Autodesk Inventor part; units mm, degrees
ref_plane "YZ Plane" through (0, 0, 0) normal (1, 0, 0) x (0, 1, 0)
ref_plane "XZ Plane" through (0, 0, 0) normal (0, 1, 0) x (-1, 0, 0)
ref_plane "XY Plane" through (0, 0, 0) normal (0, 0, 1) x (1, 0, 0)
sketch "Boceto1" plane through (0, 0, 0) normal (0, 0, 1) x (1, 0, 0)
  line L0 (2, 0) -> (4, 0)
  line L1 (6, 2) -> (6, 34)
  line L2 (3, 0) -> (3, 4)
  circle A0 centre (3, 4) radius 1
  arc A1 (6, 34) -> (0, 34) centre (3, 34) ccw
  line L3 (0, 34) -> (0, 2)
  arc A2 (0, 2) -> (2, 0) centre (2, 2) ccw
  arc A3 (4, 0) -> (6, 2) centre (4, 2) ccw
  point P0 (0, 0)
  point P1 (6, 0)
  dimension "d2" = 4
  dimension "d3" = 2
  dimension "d6" = 2
  dimension "d7" = 6
  dimension "d8" = 37
extrude "Extrusión1" add sketch "Boceto1" along normal blind 1
equation "\"thikness\" = 2"
equation "\"offset\" = 1"
equation "\"r1\" = 5.55"
equation "\"r2o\" = 59.75"
equation "\"delta_y\" = 6"
equation "\"wire_d\" = 1"
equation "\"width_ang_spring\" = 5"
equation "\"spring_int_diam\" = 8.5"
equation "\"spring_ext_diam\" = 10.5"
equation "\"r3\" = 8.25"
equation "\"r3R\" = 4.75"
equation "\"r3T\" = 6.74537"
equation "\"alpha\" = 54.847297deg"
equation "\"alpha2\" = 270deg"
equation "\"theta3_recogido\" = 305.152703deg"
equation "\"delta_theta_3\" = 45deg"
equation "\"joint_width\" = 12"
equation "\"joint_radius\" = 7.75"
equation "\"shaft_width\" = 15"
equation "\"shaft_joint_diameter\" = 7.75"
equation "\"separation_space\" = 0.5"
equation "\"height_finger\" = 42"
equation "\"cell_screw_head_diameter\" = 4"
equation "\"cell_screw_diameter\" = 2"
equation "\"cell_space\" = 2"
equation "\"cell_width\" = 6"
equation "\"cell_theta_position\" = 60deg"
equation "\"cell_thikness\" = 1"
equation "\"cell_lenght\" = 37"
equation "\"cell_z_space\" = 5"
equation "\"wire_D\" = 2.3"
equation "\"width_link\" = 8"
equation "\"Dt\" = 1.05949"
equation "\"Djoint_shaft\" = 2.3"
equation "\"shaft_x\" = 1.45"
equation "\"shaft_y\" = 6.45"
equation "\"lenght_body_link\" = 186.05"
equation "\"lenght_bar_support\" = 201.65"
equation "\"wire_spring_d\" = 1"
equation "\"spring_int_d\" = 6"
equation "\"spring_lenght\" = 28"
equation "\"trigger_offset\" = 2"
equation "\"m2_theta2o\" = 107deg"
equation "\"m2_r2\" = 28"
equation "\"e\" = 9"
equation "\"So\" = 17"
equation "\"m2_theta3o\" = -30deg"
equation "\"m2_r3\" = 19.75"
equation "\"m2_delta_theta1\" = 15deg"
equation "\"m2_theta3f\" = -60deg"
equation "\"trigger_thumb_lenght\" = 6"
equation "\"width_r12\" = 8"
equation "\"m2_r1\" = 25.2"
equation "\"r3_thikness\" = 3.5"
equation "\"t_thikness\" = 3"
equation "\"tg_width\" = 4"
equation "\"pivot_screw_d\" = 4"
equation "\"pivot_diameter\" = 7"
equation "\"sj_diam_shaft\" = 6"
equation "\"sj_groove\" = 2"
equation "\"sj_groove_deep\" = 7"
equation "\"sj_head_D\" = 7"
equation "\"sj_head_d\" = 4.7464"
equation "\"sj_head_height\" = 5"
equation "\"sf_lenght\" = 9.5"
equation "\"sf_base\" = 3"
equation "\"sf_head_height\" = 3"
equation "\"sf_head_width\" = 4.5"
equation "\"sf_head_offset\" = 0.25"
equation "\"sf_head_grip_width\" = 2"
equation "\"sf_head_angle\" = 45deg"
equation "\"sf_thikness\" = 5"
equation "\"screw_Dhead\" = 8"
equation "\"screw_d\" = 4"
equation "\"screw_lenght\" = 12"
equation "\"screwJ_base_D\" = 9"
equation "\"screwJ_top_D\" = 13"
equation "\"gj_D\" = 6"
equation "\"gj_d\" = 4"
equation "\"gj_out_section\" = 6"
equation "\"ext_width_slider\" = 3.5"
equation "\"sfbox_tip_width\" = 2.5"
equation "\"slim_width_slider\" = 1.5"
equation "\"agarradera_width\" = 4"
equation "\"int_width_slider\" = 2"
equation "\"agarradera_position\" = 82.13077"
equation "\"sfbox_theta1\" = 60deg"
equation "\"sfbox_theta2\" = 45deg"
equation "\"agarradera_theta\" = 60deg"
equation "\"sfbox_width\" = 1.5"
equation "\"box_fat_slider_lenght\" = 67"
equation "\"fat_width_slider\" = 2"
equation "\"box_in_width\" = 72"
equation "\"flex_separation_theta\" = 60deg"
equation "\"sf_flex_separation\" = 38.66667"
equation "\"thikness_box\" = 1.5"
equation "\"box_slim_slider_lenght\" = 116"
equation "\"box_in_deep\" = 77"
equation "\"box_in_height\" = 35"
properties part number "celda de carga"
Source: CAD feature listing. Evaluate the final solid. Frame: model axes, mm. Give positions to 0.01 mm unless a question says otherwise; leave off trailing zeros. Loops run counter-clockwise (first coordinate to the right, second up) from the corner with the lowest first, then second, coordinate; pieces in that order, holes last. Notation, with made-up numbers: M -20,61 L 4,61 A3 ccw 4,66 Z; hole C -16.5,-14.5 d2. An arc over 180 degrees is marked long. Put each result on its own line as item: value.
Q1. Section C-C (x = 3). Return the cut outline in (y, z).
Response values:
outline: M 0,0 L 3,0 L 3,1 L 0,1 Z; M 5,0 L 37,0 L 37,1 L 5,1 Z
Q2. Mould query, pull axis X, two halves, no side actions, for faces 1 (the flat face through (3, 19, 1)), 2 (the cylindrical face through (2.9, 37, 0.5)), 3 (the flat face through (0, 18.2, 0.5)), 4 (the cylindrical face through (2.263, 3.324, 0.493)). Classes: released by +X, released by -X, zero draft, split by the parting line, or undercut.
Response values:
face 1: zero draft
face 2: split by the parting line
face 3: released by -X
face 4: undercut
Q3. Section A-A (z = 0.2). Return the cut outline in (x, y).
Response values:
outline: M 0,2 A2 ccw 2,0 L 4,0 A2 ccw 6,2 L 6,34 A3 ccw 0,34 Z; hole C 3,4 d2
Q4. Section D-D (x = 5.6). Return the cut outline in (y, z), and give its area (3 significant figures).
Response values:
outline: M 0.8,0 L 35.5,0 L 35.5,1 L 0.8,1 Z
area: 34.7 mm²
Q5. Section B-B (y = 4). Return the cut outline in (x, z).
Response values:
outline: M 0,0 L 2,0 L 2,1 L 0,1 Z; M 4,0 L 6,0 L 6,1 L 4,1 Z
Q6. Line query: probe 1 along Y at (x, z) = (3, 0.6); probe 2 along X at (y, z) = (4, 0.3); probe 3 along Y at (x, z) = (5.2, 0.3). Output: solid intervals per line, ascending. Write a range as [from, to].
Response values:
probe 1: y = [0, 3], [5, 37]
probe 2: x = [0, 2], [4, 6]
probe 3: y = [0.4, 36.04]
